Answer from the drawing. Dimensions are ordinates in mm from the lowest x, y and z of the part. A direction names the side the tool comes from. Round coordinates to 2 decimals unless told otherwise and drop trailing zeros. Loops run counter-clockwise (first coordinate to the right, second up) from the corner with the lowest first, then second, coordinate; pieces in that order, holes last. Notation, with made-up numbers: (28, 74.25) - (36, 74.25) arc R24 ccw to (36, 92.25) - close; hole circle Ø11 at (34.5, 29.5). An arc over 180 degrees is marked (long way). Use CSV: the item, a comma, the result in double quotes. Start each with the question number.
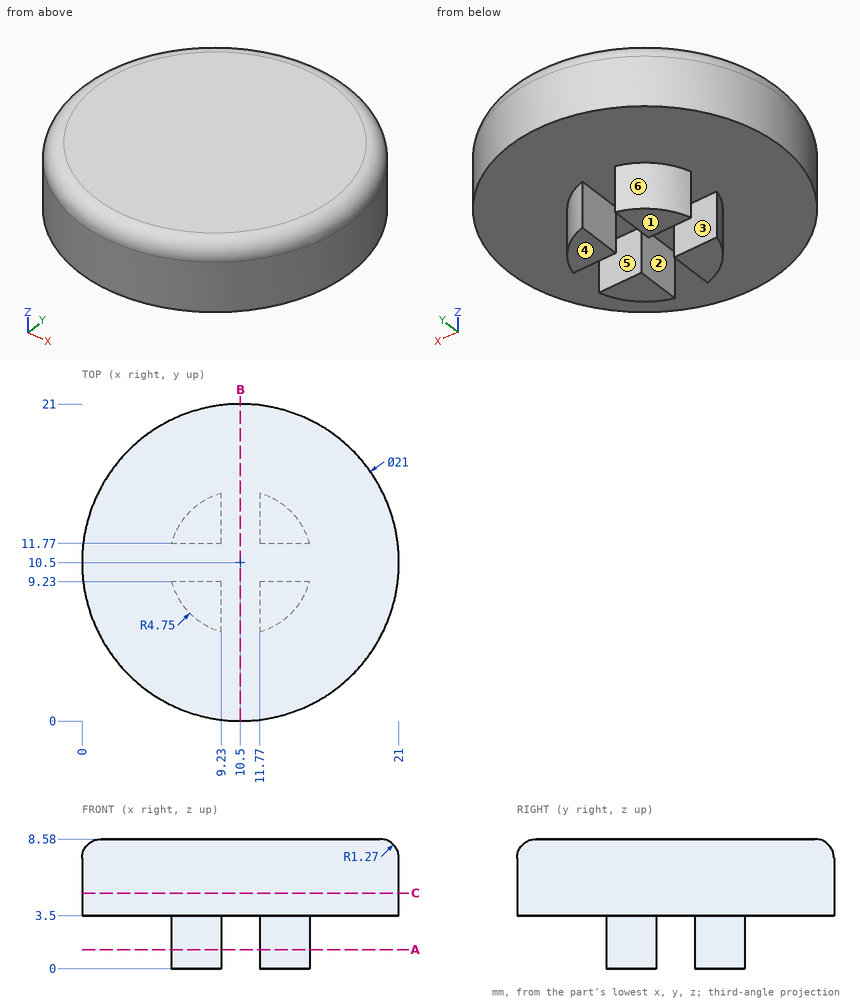
Item 1: A cutting plane is placed at C-C (z = 5). Determine the outline of the cut face in (x, y).
Item 2: Each of these flat-tipped pins is pushed along its axis until it touches: pin 1 Ø2.5 at (y, z) = (14, 1) entering from +X; pin 2 Ø1.5 at (x, z) = (8, 2.5) entering from -Y; pin 3 Ø1 at (x, z) = (7, 1.5) entering from -Y. Where does it stop, or does it pass through?
Item 3: A cutting plane is placed at A-A (z = 1.25). Determine the outline of the cut face in (x, y).
Item 4: A cutting plane is placed at B-B (x = 10.5). Determine the outline of the cut face in (y, z).
Item 5: The mould has two halves that part along Y. Classify the marked faces 3, 4, 5 and 6: pulls with the +Y half, pulls with the -Y half, needs draft (parallel to the pull), parting line crosses it, or undercut.
Item 6: Find the intervals of material crossed by probe 1 along Z at (x, y) = (18.5, 6.75); probe 2 along Y at (x, z) = (8.75, 1); probe 3 along Y at (x, z) = (10.5, 6), in increasing order. Write a range as [from, to].
Item 7: Which of the six approach directions +Z, -Z, +X, -X, +Y, -Y give full straight-line access (tool end or side, diameter ignored) to the marked faces 1 and 2?
Result sheet:
1,outline,"circle Ø21 at (10.5, 10.5)"
2,pin 1,"x = 14.68"
2,pin 2,"y = 6.08"
2,pin 3,"y = 6.82"
3,outline,"(5.92, 9.23) arc R4.75 ccw to (9.23, 5.92) - (9.23, 9.23) - close; (5.92, 11.77) - (9.23, 11.77) - (9.23, 15.08) arc R4.75 ccw to start; (11.77, 5.92) arc R4.75 ccw to (15.08, 9.23) - (11.77, 9.23) - close; (11.77, 11.77) - (15.08, 11.77) arc R4.75 ccw to (11.77, 15.08) - close"
4,outline,"(0, 3.5) - (21, 3.5) - (21, 7.31) arc R1.27 ccw to (19.73, 8.58) - (1.27, 8.58) arc R1.27 ccw to (0, 7.31) - close"
5,face 3,"undercut"
5,face 4,"needs draft"
5,face 5,"undercut"
5,face 6,"pulls with the +Y half"
6,probe 1,"[3.5, 8.58]"
6,probe 2,"[6.08, 9.23], [11.77, 14.92]"
6,probe 3,"[0, 21]"
7,face 1,"-Z, +X, -X, +Y, -Y"
7,face 2,"-Z, +Y, -Y"
